from build123d import *

# Parameters (mm, degrees)
SKETCH1_W                    = 105
SKETCH1_H                    = 725.7
BASE_FLANGE1_DEPTH           = 1
EDGE_FLANGE1_STRIP_W         = 6
EDGE_FLANGE1_STRIP_H         = 1
EDGE_FLANGE1_STRIP_CUT_DEPTH = 725.7
EDGE_FLANGE1_DEPTH           = 725.7
EDGE_FLANGE2_STRIP_W         = 6
EDGE_FLANGE2_STRIP_H         = 1
EDGE_FLANGE2_STRIP_CUT_DEPTH = 725.7
EDGE_FLANGE2_DEPTH           = 725.7
SKETCH19_R                   = 2.5
CUT_EXTRUDE2_DEPTH           = 10
CUT_EXTRUDE3_START           = -20.5
CUT_EXTRUDE3_DEPTH           = 20.5


# Read off the part's stored shape, not the designer's step: Cut-Extrude3
# Sheet-metal steps are written as plain solids
with BuildPart() as part:
    # Sketch1 → Base-Flange1 (new body)
    with BuildSketch(Plane(origin=(0, 0, 0), x_dir=(1, 0, 0), z_dir=(0, 1, 0))):
        with Locations((52.5, 362.85)):
            Rectangle(SKETCH1_W, SKETCH1_H)
    extrude(amount=-BASE_FLANGE1_DEPTH)

    # Edge-Flange1 strip (across the edge) → Edge-Flange1 strip cut (cut)
    with BuildSketch(Plane(origin=(105, 0, 0), x_dir=(-1, 0, 0), z_dir=(0, 0, -1))):
        with Locations((-1, -0.5)):
            Rectangle(EDGE_FLANGE1_STRIP_W, EDGE_FLANGE1_STRIP_H)
    extrude(amount=EDGE_FLANGE1_STRIP_CUT_DEPTH, mode=Mode.SUBTRACT)

    # Edge-Flange1 section (across the edge) → Edge-Flange1 (add)
    with BuildSketch(Plane(origin=(105, 0, 0), x_dir=(-1, 0, 0), z_dir=(0, 0, -1))):
        with BuildLine():
            Line((0, 1), (0, 19))
            Line((0, 19), (1, 19))
            Line((1, 19), (1, 1))
            ThreePointArc((1, 1), (1.292893219, 0.292893219), (2, 0))
            Line((2, 0), (2, -1))
            ThreePointArc((2, -1), (0.585786438, -0.414213562), (0, 1))
        make_face()
    extrude(amount=EDGE_FLANGE1_DEPTH)

    # Edge-Flange2 strip (across the edge) → Edge-Flange2 strip cut (cut)
    with BuildSketch(Plane(origin=(104, 19, 0), x_dir=(0, -1, 0), z_dir=(0, 0, -1))):
        with Locations((-1, -0.5)):
            Rectangle(EDGE_FLANGE2_STRIP_W, EDGE_FLANGE2_STRIP_H)
    extrude(amount=EDGE_FLANGE2_STRIP_CUT_DEPTH, mode=Mode.SUBTRACT)

    # Edge-Flange2 section (across the edge) → Edge-Flange2 (add)
    with BuildSketch(Plane(origin=(104, 19, 0), x_dir=(0, -1, 0), z_dir=(0, 0, -1))):
        with BuildLine():
            Line((0, 1), (0, 12))
            Line((0, 12), (1, 12))
            Line((1, 12), (1, 1))
            ThreePointArc((1, 1), (1.292893219, 0.292893219), (2, 0))
            Line((2, 0), (2, -1))
            ThreePointArc((2, -1), (0.585786438, -0.414213562), (0, 1))
        make_face()
    extrude(amount=EDGE_FLANGE2_DEPTH)

    # Sketch19 → Cut-Extrude2 (cut)
    with BuildSketch(Plane(origin=(0, 19, 0), x_dir=(1, 0, 0), z_dir=(0, 1, 0))):
        with Locations(Location((98, 662.7, 0), (0, 0, 180))):
            Circle(SKETCH19_R)
        with Locations(Location((98, 617.7, 0), (0, 0, 180))):
            Circle(SKETCH19_R)
        with Locations(Location((98, 449.7, 0), (0, 0, 180))):
            Circle(SKETCH19_R)
        with Locations(Location((98, 281.7, 0), (0, 0, 180))):
            Circle(SKETCH19_R)
        with Locations(Location((98, 113.7, 0), (0, 0, 180))):
            Circle(SKETCH19_R)
        with Locations((98, -54.3)):
            Circle(SKETCH19_R)
    extrude(amount=-CUT_EXTRUDE2_DEPTH, mode=Mode.SUBTRACT)

    # Cut-Extrude3 outline → Cut-Extrude3 (cut)
    with BuildSketch(Plane.XY.offset(CUT_EXTRUDE3_START)):
        with BuildLine():
            ThreePointArc((104, 1), (103.707106781, 0.292893219), (103, 0))
            Line((103, 0), (103, -1))
            ThreePointArc((103, -1), (104.414213562, -0.414213562), (105, 1))
            Line((105, 1), (105, 17))
            ThreePointArc((105, 17), (104.414213562, 18.414213562), (103, 19))
            Line((103, 19), (92, 19))
            Line((92, 19), (92, 18))
            Line((92, 18), (103, 18))
            ThreePointArc((103, 18), (103.707106781, 17.707106781), (104, 17))
            Line((104, 17), (104, 1))
        make_face()
    extrude(amount=CUT_EXTRUDE3_DEPTH, mode=Mode.SUBTRACT)


solid = part.part
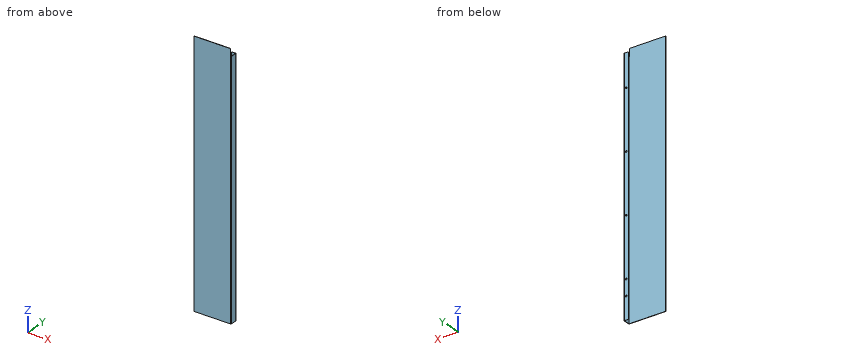
CAD build for the part. Positions are in the model's coordinates, mm. Round coordinates to 2 decimals unless told otherwise and drop trailing zeros. Write each loop counter-clockwise with the first axis right and the second up, starting at its lowest first coordinate (ties: lowest second). Pieces come first, ordered by that corner, then holes.
(1) Slice it at C-C, the plane y = 9.25. Write the cut outline in (x, z).
(2) Probe line 1 along Z through (x, y) = (98, 18.25); line 2 along Y through (x, z) = (95.5, -452); line 3 along X through (y, z) = (18.7, -662.7). List the from-to ranges inside material, lowest first.
(3) Drop flat-ended pins along their axis: P1, Ø3, axis at x = 20, z = -409, coming from the +Y side; P2, Ø5, axis at y = 8.5, z = -429.5, coming from the -X side; P3, Ø1.1, axis at y = -0.5, z = -12.5, coming from the +X side. Give the stop position or say it passes through.
(4) Slice it at A-A, the plane z = -344. Write the cut outline in (x, y), and give its area (3 significant figures).
(5) Slice it at B-B, the plane x = 29. Write the cut outline in (y, z), and give its area (3 significant figures).
From the geometry:
1. outline: (104, -725.7) - (105, -725.7) - (105, -20.5) - (104, -20.5) - close
2. line 1: z = -725.7 to -665.2, -660.2 to -620.2, -615.2 to -452.2, -447.2 to -284.2, -279.2 to -116.2, -111.2 to -20.5
2. line 2: y = -1 to 0, 18 to 19
2. line 3: x = 92 to 95.5, 100.5 to 104.05
3. P1: stops at y = 0
3. P2: stops at x = 104
3. P3: stops at x = 103
4. outline: (0, -1) - (103, -1) arc R2 ccw to (105, 1) - (105, 17) arc R2 ccw to (103, 19) - (92, 19) - (92, 18) - (103, 18) arc R1 cw to (104, 17) - (104, 1) arc R1 cw to (103, 0) - (0, 0) - close
4. area: 135 mm2
5. outline: (-1, -725.7) - (0, -725.7) - (0, 0) - (-1, 0) - close
5. area: 726 mm2
